```python
from build123d import *

# Parameters (mm, degrees)
SKETCH_1_R          = 40
EXTRUDE_1_DEPTH     = 5
SKETCH_2_R          = 5
EXTRUDE_2_DEPTH     = 15
SKETCH_3_R          = 40
EXTRUDE_3_DEPTH     = 5
SKETCH_4_R          = 5
EXTRUDE_4_DEPTH     = 15
SKETCH_5_R          = 40
EXTRUDE_5_DEPTH     = 5
SKETCH_6_R          = 20
EXTRUDE_6_DEPTH     = 35
SKETCH_7_R          = 14
CUT_EXTRUDE_1_DEPTH = 57
CUT_EXTRUDE_2_DEPTH = 57


with BuildPart() as part:
    # 草图1 → 凸台-拉伸1 (new body)
    with BuildSketch(Plane.XY):
        Circle(SKETCH_1_R)
    extrude(amount=EXTRUDE_1_DEPTH)

    # 草图2 → 凸台-拉伸2 (add)
    with BuildSketch(Plane.XY.offset(5)):
        with Locations((32, 0)):
            Circle(SKETCH_2_R)
        with Locations((0, -32)):
            Circle(SKETCH_2_R)
        with Locations((-32, 0)):
            Circle(SKETCH_2_R)
        with Locations((0, 32)):
            Circle(SKETCH_2_R)
    extrude(amount=EXTRUDE_2_DEPTH)

    # 草图3 → 凸台-拉伸3 (add)
    with BuildSketch(Plane.XY.offset(20)):
        Circle(SKETCH_3_R)
    extrude(amount=EXTRUDE_3_DEPTH)

    # 草图4 → 凸台-拉伸4 (add)
    with BuildSketch(Plane.XY.offset(25)):
        with Locations((22.627416998, -22.627416998)):
            Circle(SKETCH_4_R)
        with Locations((-22.627416998, -22.627416998)):
            Circle(SKETCH_4_R)
        with Locations((-22.627416998, 22.627416998)):
            Circle(SKETCH_4_R)
        with Locations((22.627416998, 22.627416998)):
            Circle(SKETCH_4_R)
    extrude(amount=EXTRUDE_4_DEPTH)

    # 草图5 → 凸台-拉伸5 (add)
    with BuildSketch(Plane.XY.offset(40)):
        Circle(SKETCH_5_R)
    extrude(amount=EXTRUDE_5_DEPTH)

    # 草图6 → 凸台-拉伸6 (add)
    with BuildSketch(Plane.XY.offset(5)):
        Circle(SKETCH_6_R)
    extrude(amount=EXTRUDE_6_DEPTH)

    # 草图7 → 切除-拉伸1 (cut)
    with BuildSketch(Plane.XY.offset(45)):
        Circle(SKETCH_7_R)
    extrude(amount=-CUT_EXTRUDE_1_DEPTH, mode=Mode.SUBTRACT)

    # 草图8 → 切除-拉伸2 (cut)
    with BuildSketch(Plane.XY.offset(45)):
        Polygon((-4, 14), (-4, 9.394877301), (4, 9.394877301), (4, 14), (4, 17.2), (-4, 17.2), align=None)
    extrude(amount=-CUT_EXTRUDE_2_DEPTH, mode=Mode.SUBTRACT)


solid = part.part
```
Geometry: final body of the model. Coordinates: model frame, mm. A direction names the side the tool comes from. Coordinates: 2 decimals unless noted, no trailing zeros. Order: outer loops, then holes, each group sorted by start corner. A loop starts at its lowest first (then second) coordinate and runs counter-clockwise, first axis right, second up. Notation, with made-up numbers: (18.5, 50.5) - (67.5, 50.5) arc R20 cw to (67.5, 63.5) - close; hole circle Ø2 at (-17, 0.5). An arc over 180 degrees is marked (long way). Write each question's results on one line, items separated by ' | '.
(1) Section query C-C, the plane x = 32. Return the cut outline in (y, z), plus the area to 3 significant figures.
Values found:
outline: (-24, 0) - (24, 0) - (24, 5) - (5, 5) - (5, 20) - (24, 20) - (24, 25) - (-24, 25) - (-24, 20) - (-5, 20) - (-5, 5) - (-24, 5) - close; (-24, 40) - (24, 40) - (24, 45) - (-24, 45) - close | area: 870 mm²
(2) Section query B-B, the plane x = 0. Count the separate pieces of the cut face and the enclosed holes in it, plus the area to 3 significant figures.
Values found:
separate pieces: 2 | enclosed holes: 2 | area: 1,300 mm²
(3) Line query: line 1 (Y direction, x = 0, z = 15); line 2 (Z direction, x = 33, y = 19); line 3 (Y direction, x = 0, z = 26). Output: solid intervals per line, ascending. Write a range as [from, to].
Values found:
line 1: y = [-37, -27], [-20, -14], [17.2, 20], [27, 37] | line 2: z = [0, 5], [20, 25], [40, 45] | line 3: y = [-20, -14], [17.2, 20]
(4) Set-up query: faces 1 (the face through (0, 17.2, 23)), 2 (the face through (27.4, -21.13, 32.39)). Return all of +Z, -Z, +X, -X, +Y, -Y with unobstructed straight access to the full face (end or side cutting, diameter ignored); none if empty.
Values found:
face 1: +Z, -Z | face 2: none
(5) Mould query, pull axis X, two halves, no side actions, for faces 3 (the face through (-9.4, 18.3, 25)), 4 (the face through (-9.4, 18.3, 40)), 5 (the face through (-1, -17, 0)), 6 (the face through (-8.67, -39.05, 2.46)). Classes: +X half, -X half, draft (parallel to the pull), parting line (faces both ways), or undercut.
Values found:
face 3: undercut | face 4: undercut | face 5: draft | face 6: parting line
(6) Section query A-A, the plane z = 12.5. Return the cut outline in (x, y), plus the area to 3 significant figures.
Values found:
outline: circle Ø10 at (-32, 0); circle Ø40 at (0, 0); circle Ø10 at (0, -32); circle Ø10 at (0, 32); circle Ø10 at (32, 0); hole (-4, 13.42) arc R14 ccw (long way) to (4, 13.42) - (4, 17.2) - (-4, 17.2) - close | area: 928 mm²
(7) First-contact query: pin 1 Ø6.5 at (x, z) = (2, 31) entering from -Y; pin 2 Ø4 at (y, z) = (15, 20) entering from -X; pin 3 Ø8 at (x, z) = (-12, 34.5) entering from -Y; pin 4 Ø24 at (x, y) = (19, -8.5) entering from -Z. Flat tips, straight axial feed; report the tip coordinate or a pass-through.
Values found:
pin 1: stops at y = -20 | pin 2: stops at x = -37.83 | pin 3: stops at y = -18.33 | pin 4: stops at z = 0
